The listing builds one solid part. Answer for the finished solid, in the listing's coordinates (mm). A direction names the side the tool comes from. Round coordinates to 2 decimals unless told otherwise and drop trailing zeros. Order: outer loops, then holes, each group sorted by start corner. A loop starts at its lowest first (then second) coordinate and runs counter-clockwise, first axis right, second up. Notation, with made-up numbers: (45.5, 10) - (53.5, 10) arc R26 cw to (53.5, 41) - close; hole circle Ø5 at (65, 6). An arc over 180 degrees is marked (long way). One line per item, written item: value. Start each with the question number.
1. Straight lines are drawn through the part: line 1 (Y direction, x = -22.2, z = -14); line 2 (Z direction, x = -18, y = 33); line 3 (X direction, y = 18, z = -8). For each, find the intervals that lie inside material, in ascending order.
2. Flat-ended cylindrical pins translate along their axes: P1, Ø2.5, axis at x = -18, z = -4.5, coming from the -Y side; P2, Ø5.5, axis at y = 39.5, z = 0, coming from the -X side; P3, Ø17.5, axis at x = -7, z = -4, coming from the +Y side. Find the tip coordinate at first contact, or state that the pin passes through.
3. Section B-B, the plane x = 17 is taken. Give the vertices of the cut face in (y, z), then the cut area to 3 significant figures.
4. Section A-A, the plane y = 39.5 is taken. Give the vertices of the cut face in (x, z).
5. Section C-C, the plane z = -14 is taken. Give the vertices of the cut face in (x, y).
6. A tool of negligible diameter and unlimited length cuts with its end or side. For faces 1 (the flat face through (0.3, 0, 4.3)), 2 (the flat face through (22, 25, 0)), 3 (the cylindrical face through (-22.25, 32.66, -13.46)), from which of +Z, -Z, +X, -X, +Y, -Y can it reach the whole face along a straight path? Write none if from no direction.
7. For a pull along X with two mould halves and no side action, classify faces 4 (the flat face through (0, 25, 17.5)), 5 (the cylindrical face through (-22.246, 36.526, -0.391)), 6 (the cylindrical face through (3.905, 1.232, -0.867)), 7 (the flat face through (22.5, 23, 0)) as released by +X, released by -X, zero draft, split by the parting line, or undercut.
8. Section D-D, the plane y = 33.5 is taken. Give the vertices of the cut face in (x, z).
Autodesk Inventor part; units mm, degrees
ref_plane "YZ Plane" through (0, 0, 0) normal (1, 0, 0) x (0, 1, 0)
ref_plane "XZ Plane" through (0, 0, 0) normal (0, 1, 0) x (-1, 0, 0)
ref_plane "XY Plane" through (0, 0, 0) normal (0, 0, 1) x (1, 0, 0)
sketch "Sketch1" plane through (0, 0, 0) normal (0, 1, 0) x (-1, 0, 0)
  line L0 (-22.5, 18) -> (22.5, 18)
  line L1 (22.5, 18) -> (22.5, -18)
  line L2 (22.5, -18) -> (-22.5, -18)
  line L3 (-22.5, -18) -> (-22.5, 18)
  line L4 (-22.5, 18) -> (22.5, -18) construction
  line L5 (22.5, 18) -> (-22.5, -18) construction
  line L6 (-22, 17.5) -> (22, 17.5)
  line L7 (22, 17.5) -> (22, -17.5)
  line L8 (22, -17.5) -> (-22, -17.5)
  line L9 (-22, -17.5) -> (-22, 17.5)
  line L10 (-22, 17.5) -> (22, -17.5) construction
  line L11 (22, 17.5) -> (-22, -17.5) construction
  point P0 (0, 0)
  dimension "d0" = 45
  dimension "d1" = 36
  dimension "d2" = 44
  dimension "d3" = 35
extrude "Extrusion1" add sketch "Sketch1" along normal blind 2.5 contours L6 L7 L8 L9
extrude "Extrusion2" add sketch "Sketch1" along normal blind 47.5
sketch "Sketch2" plane through (0, 2.5, 0) normal (0, 1, 0) x (1, 0, 0)
  line L0 (-22.5, 18) -> (-22.5, -18)
  line L1 (22.5, 18) -> (-22.5, 18)
  line L2 (-22.5, 18) -> (-22.5, -18)
  line L3 (-22.5, -18) -> (22.5, -18)
  line L4 (22.5, -18) -> (22.5, 18)
  line L5 (22.5, 18) -> (-22.5, -18) construction
  line L6 (-22.5, 18) -> (22.5, -18) construction
  line L7 (22.5, 18) -> (-22.5, 18)
  line L8 (-22.5, 18) -> (-22.5, 13.5)
  line L9 (-22.5, 13.5) -> (-18, 13.5)
  line L10 (-18, 13.5) -> (-18, 4.5)
  point P0 (0, 0)
  point P1 (0, 0)
  dimension "d8" = 4.5
  dimension "d9" = 4.5
  dimension "d10" = 9
hole "Hole1" at (-18, 2.5, -4.5) at (-18, 2.5, -13.5) direction (0, -1, 0) diameter 3 depth 8
hole "Hole2" at (0, 2.5, 0) direction (0, -1, 0) diameter 8 depth 8
sketch "Sketch3" plane through (-22.5, 0, -18) normal (-1, 0, 0) x (0, 0, 1)
  line L0 (0, 0) -> (36, 0)
  line L1 (36, 0) -> (36, 47.5)
  line L2 (0, 47.5) -> (36, 47.5)
  line L3 (0, 0) -> (0, 47.5)
  line L4 (0, 47.5) -> (18, 47.5)
  line L5 (0, 47.5) -> (36, 47.5)
  line L6 (18, 47.5) -> (18, 39.5)
  line L7 (18, 39.5) -> (4, 39.5)
  line L8 (4, 39.5) -> (4, 33.5)
  point P0 (18, 0)
  dimension "d25" = 18
  dimension "d26" = 8
  dimension "d27" = 14
  dimension "d28" = 6
hole "Hole3" at (-22.5, 33.5, -14) at (-22.5, 39.5, -14) direction (1, 0, 0) diameter 2 depth 8
hole "Hole4" at (-22.5, 39.5, 0) direction (1, 0, 0) diameter 6 depth 8
thread "Thread1"
thread "Thread2"
properties part number "HUDISN-1-53"
Answer list:
1. line 1: y = 0 to 32.5, 34.5 to 38.5, 40.5 to 47.5
1. line 2: z = -18 to -17.5, 17.5 to 18
1. line 3: x = -22.5 to -22, 22 to 22.5
2. P1: passes through
2. P2: stops at x = 22
2. P3: stops at y = 2.5
3. outline: (0, -18) - (47.5, -18) - (47.5, -17.5) - (2.5, -17.5) - (2.5, 17.5) - (47.5, 17.5) - (47.5, 18) - (0, 18) - close
3. area: 135 mm²
4. outline: (-22.5, -18) - (22.5, -18) - (22.5, 18) - (-22.5, 18) - (-22.5, 3) - (-22, 3) - (-22, 17.5) - (22, 17.5) - (22, -17.5) - (-22, -17.5) - (-22, -15) - (-22.5, -15) - close; (-22.5, -13) - (-22, -13) - (-22, -3) - (-22.5, -3) - close
5. outline: (-22.5, 0) - (-19.41, 0) - (-19.41, 2.5) - (-22, 2.5) - (-22, 32.5) - (-22.5, 32.5) - close; (-22.5, 34.5) - (-22, 34.5) - (-22, 38.5) - (-22.5, 38.5) - close; (-22.5, 40.5) - (-22, 40.5) - (-22, 47.5) - (-22.5, 47.5) - close; (-16.59, 0) - (22.5, 0) - (22.5, 47.5) - (22, 47.5) - (22, 2.5) - (-16.59, 2.5) - close
6. face 1: +Z, -Z, +X, -X, -Y
6. face 2: +Y
6. face 3: -X
7. face 4: undercut
7. face 5: zero draft
7. face 6: undercut
7. face 7: released by +X
8. outline: (-22.5, -18) - (22.5, -18) - (22.5, 18) - (-22.5, 18) - (-22.5, -13) - (-22, -13) - (-22, 17.5) - (22, 17.5) - (22, -17.5) - (-22, -17.5) - (-22, -15) - (-22.5, -15) - close
